Job drawing, mm, ordinate dimensions from the low corner. One solid piece. A direction names the side the tool comes from. Round coordinates to 2 decimals unless told otherwise and drop trailing zeros. Order: outer loops, then holes, each group sorted by start corner. A loop starts at its lowest first (then second) coordinate and runs counter-clockwise, first axis right, second up. Notation, with made-up numbers: M -5.75,19.25 L 50.25,19.25 A22 ccw 50.25,57.25 Z; hole C -33,57 d4. An arc over 180 degrees is marked long. Answer as a JSON object with one key per item and string values. Group by question number.
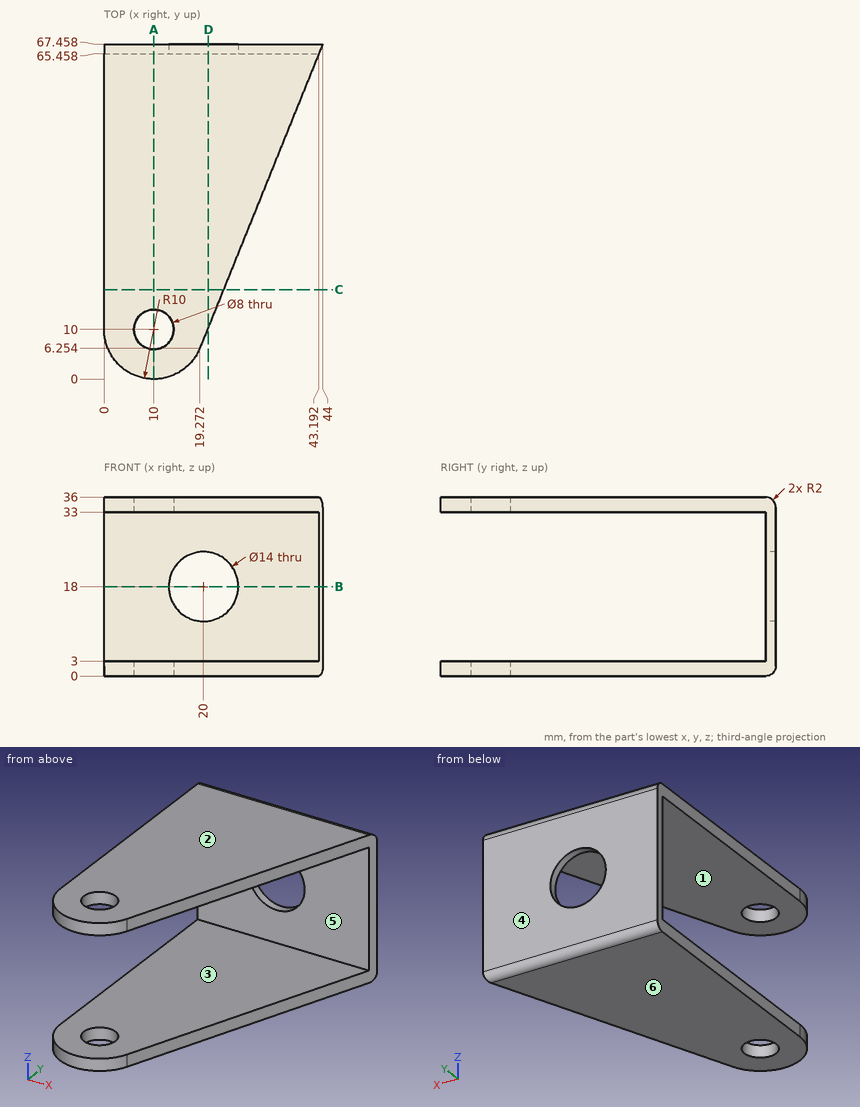
Item 1: Drill centre lines: line 1 (Y direction, x = 10, z = 34); line 2 (Z direction, x = 15.5, y = 4); line 3 (Y direction, x = 8, z = 20.5). Where is each one in solid material? Low to high. Write a range as [from, to].
Item 2: Cut at C-C, the plane y = 18. Give the cut face in (x, z).
Item 3: Flat gauge pins, fed straight in: pin 1 Ø1 at (x, z) = (13, 16.5) entering from -Y; pin 2 Ø6 at (y, z) = (30.5, 31.5) entering from +X; pin 3 Ø12.5 at (x, z) = (20, 18) entering from -Y; pin 4 Ø10 at (y, z) = (59.5, 31) entering from +X. Where does each tip first touch, or does it go through?
Item 4: 3-axis set-ups, long thin cutter, end or side, ignore diameter. For the marked faces 5 and 6: which of +Z, -Z, +X, -X, +Y, -Y reach the whole face in a straight line?
Item 5: Cut at A-A, the plane x = 10. Give the cut face in (y, z).
Item 6: Two-plate mould, pull along Z, no slides. Class the marked faces 1, 2, 3 and 4: +Z half, -Z half, draft (parallel to the pull), parting line (faces both ways), or undercut.
Item 7: Cut at D-D, the plane x = 21. Give the cut face in (y, z), and give its area (3 significant figures).
Item 8: Cut at B-B, the plane z = 18. Give the cut face in (x, y).
Response values:
{
 "1": {"line 1": "[0, 6], [14, 67.46]", "line 2": "[0, 3], [33, 36]", "line 3": "[65.46, 67.46]"},
 "2": {"outline": "M 0,0 L 24.02,0 L 24.02,3 L 0,3 Z; M 0,33 L 24.02,33 L 24.02,36 L 0,36 Z"},
 "3": {"pin 1": "y = 65.46", "pin 2": "x = 30.12", "pin 3": "through", "pin 4": "x = 42.64"},
 "4": {"face 5": "+X, -X, -Y", "face 6": "-Z, +X, -X, +Y, -Y"},
 "5": {"outline": "M 0,0 L 6,0 L 6,3 L 0,3 Z; M 0,33 L 6,33 L 6,36 L 0,36 Z; M 14,0 L 65.46,0 A2 ccw 67.46,2 L 67.46,34 A2 ccw 65.46,36 L 14,36 L 14,33 L 65.46,33 L 65.46,3 L 14,3 Z"},
 "6": {"face 1": "undercut", "face 2": "+Z half", "face 3": "undercut", "face 4": "draft"},
 "7": {"outline": "M 10.53,0 L 65.46,0 A2 ccw 67.46,2 L 67.46,11.07 L 65.46,11.07 L 65.46,3 L 10.53,3 Z; M 10.53,33 L 65.46,33 L 65.46,24.93 L 67.46,24.93 L 67.46,34 A2 ccw 65.46,36 L 10.53,36 Z", "area": "372 mm^2"},
 "8": {"outline": "M 0,65.46 L 13,65.46 L 13,67.46 L 0,67.46 Z; M 27,65.46 L 43.19,65.46 L 44,67.46 L 27,67.46 Z"}
}
